Check sheet for the modelled part. Datum: model origin and axes. Units: mm. A direction names the side the tool comes from. Coordinates: 2 decimals unless noted, no trailing zeros. Loops run counter-clockwise (first coordinate to the right, second up) from the corner with the lowest first, then second, coordinate; pieces in that order, holes last.
```python
from build123d import *

# Parameters (mm, degrees)
BOSS_EXTRUDE1_DEPTH   = 7.2
SKETCH1_3_R           = 3.75
SKETCH1_3_R_2         = 1.6
BOSS_EXTRUDE2_DEPTH   = 2
BOSS_EXTRUDE2_2_DEPTH = 2
BOSS_EXTRUDE3_DEPTH   = 2
BOSS_EXTRUDE4_DEPTH   = 7.5
SKETCH3_R             = 3.75
CUT_EXTRUDE6_DEPTH    = 12
BOSS_EXTRUDE5_DEPTH   = 7.5
SKETCH5_R             = 3.75
CUT_EXTRUDE7_DEPTH    = 7.5
SKETCH6_W             = 29.5
SKETCH6_H             = 8.4
BOSS_EXTRUDE6_DEPTH   = 4.3
SKETCH7_W             = 7.5
SKETCH7_H             = 7.2
SKETCH7_W_2           = 16.3
BOSS_EXTRUDE7_DEPTH   = 2
SKETCH8_W             = 10.1
SKETCH8_H             = 2.3
CUT_EXTRUDE8_DEPTH    = 12
SKETCH9_W             = 10.1
SKETCH9_H             = 1.2
BOSS_EXTRUDE8_DEPTH   = 6.4
SKETCH11_W            = 9.1347476
SKETCH11_H            = 5.173710516
BOSS_EXTRUDE11_DEPTH  = 5.5
SKETCH12_R            = 3.106234899
CUT_EXTRUDE10_DEPTH   = 1.5
CUT_EXTRUDE10_DRAFT   = -25
SKETCH13_R            = 3.196774454
CUT_EXTRUDE11_DEPTH   = 1.5
CUT_EXTRUDE11_DRAFT   = -29
SKETCH14_W            = 8.1347476
SKETCH14_H            = 4.5
CUT_EXTRUDE12_DEPTH   = 4.5


# Read off the part's stored shape, not the designer's step: Dome1, Dome2
with BuildPart() as part:
    # Sketch1 → Boss-Extrude1 (new body)
    with BuildSketch(Plane(origin=(0, 0, 0), x_dir=(1, 0, 0), z_dir=(0, 1, 0))):
        Polygon((14.75, 0), (-14.75, 0), (-14.75, -3.75), (-14.75, -6.5), (14.75, -6.5), (14.75, -3.75), align=None)
        Polygon((-14.75, 3.75), (-14.75, 0), (14.75, 0), (14.75, 3.75), (14.75, 6.5), (-14.75, 6.5), align=None)
    extrude(amount=BOSS_EXTRUDE1_DEPTH)



with BuildPart() as body_2:
    # Sketch1<3> → Boss-Extrude2 (new body)
    with BuildSketch(Plane(origin=(0, 0, 0), x_dir=(1, 0, 0), z_dir=(0, 1, 0))):
        with Locations(Location((-18.5, 0, 0), (0, 0, 270))):
            Circle(SKETCH1_3_R)
        with Locations(Location((-18.5, 0, 0), (0, 0, 270))):
            Circle(SKETCH1_3_R_2, mode=Mode.SUBTRACT)
    extrude(amount=BOSS_EXTRUDE2_DEPTH)


with BuildPart() as body_3:
    # Sketch1<3> → Boss-Extrude2 2 (new body)
    with BuildSketch(Plane(origin=(0, 0, 0), x_dir=(1, 0, 0), z_dir=(0, 1, 0))):
        with Locations(Location((18.5, 0, 0), (0, 0, 270))):
            Circle(SKETCH1_3_R)
        with Locations(Location((18.5, 0, 0), (0, 0, 270))):
            Circle(SKETCH1_3_R_2, mode=Mode.SUBTRACT)
    extrude(amount=BOSS_EXTRUDE2_2_DEPTH)


with BuildPart() as part_1:
    add(part.part)

    add(body_2.part)  # Boss-Extrude3 merges body 2

    add(body_3.part)  # Boss-Extrude3 merges body 3
    # Sketch1<4> → Boss-Extrude3 (add)
    with BuildSketch(Plane(origin=(0, 0, 0), x_dir=(1, 0, 0), z_dir=(0, 1, 0))):
        with BuildLine():
            Line((-14.75, -3.75), (-14.75, 0))
            ThreePointArc((-14.75, 0), (-15.848349571, -2.651650429), (-18.5, -3.75))
            Line((-18.5, -3.75), (-14.75, -3.75))
        make_face()
        with BuildLine():
            Line((-14.75, 0), (-14.75, 3.75))
            Line((-14.75, 3.75), (-18.5, 3.75))
            ThreePointArc((-18.5, 3.75), (-15.848349571, 2.651650429), (-14.75, 0))
        make_face()
        with BuildLine():
            Line((18.5, 3.75), (14.75, 3.75))
            Line((14.75, 3.75), (14.75, 0))
            ThreePointArc((14.75, 0), (15.848349571, 2.651650429), (18.5, 3.75))
        make_face()
        with BuildLine():
            ThreePointArc((18.5, -3.75), (15.848349571, -2.651650429), (14.75, 0))
            Line((14.75, 0), (14.75, -3.75))
            Line((14.75, -3.75), (18.5, -3.75))
        make_face()
    extrude(amount=BOSS_EXTRUDE3_DEPTH)

    # Sketch2 → Boss-Extrude4 (add)
    with BuildSketch(Plane.XY.offset(3.75)):
        Polygon((18.5, 2), (14.75, 2), (14.75, 5.75), align=None)
    extrude(amount=-BOSS_EXTRUDE4_DEPTH)

    # Sketch3 → Cut-Extrude6 (cut)
    with BuildSketch(Plane(origin=(0, 2, 0), x_dir=(1, 0, 0), z_dir=(0, 1, 0))):
        with Locations((18.5, 0)):
            Circle(SKETCH3_R)
    extrude(amount=CUT_EXTRUDE6_DEPTH, mode=Mode.SUBTRACT)

    # Sketch4 → Boss-Extrude5 (add)
    with BuildSketch(Plane.XY.offset(3.75)):
        Polygon((-14.75, 5.75), (-18.5, 2), (-14.75, 2), align=None)
    extrude(amount=-BOSS_EXTRUDE5_DEPTH)

    # Sketch5 → Cut-Extrude7 (cut)
    with BuildSketch(Plane(origin=(0, 2, 0), x_dir=(1, 0, 0), z_dir=(0, 1, 0))):
        with Locations((-18.5, 0)):
            Circle(SKETCH5_R)
    extrude(amount=CUT_EXTRUDE7_DEPTH, mode=Mode.SUBTRACT)

    # Sketch6 → Boss-Extrude6 (add)
    with BuildSketch(Plane(origin=(0, 7.2, 0), x_dir=(1, 0, 0), z_dir=(0, 1, 0))):
        Rectangle(SKETCH6_W, SKETCH6_H)
    extrude(amount=BOSS_EXTRUDE6_DEPTH)

    # Sketch7 → Boss-Extrude7 (add)
    with BuildSketch(Plane(origin=(0, 11.5, 0), x_dir=(1, 0, 0), z_dir=(0, 1, 0))):
        with Locations((-10.25, 0)):
            Rectangle(SKETCH7_W, SKETCH7_H)
        with Locations((5.8, 0)):
            Rectangle(SKETCH7_W_2, SKETCH7_H)
    extrude(amount=BOSS_EXTRUDE7_DEPTH)

    # Sketch8 → Cut-Extrude8 (cut)
    with BuildSketch(Plane(origin=(0, 7.2, 0), x_dir=(1, 0, 0), z_dir=(0, 1, 0))):
        with Locations((0.003829246, -5.35)):
            Rectangle(SKETCH8_W, SKETCH8_H)
    extrude(amount=-CUT_EXTRUDE8_DEPTH, mode=Mode.SUBTRACT)

    # Sketch9 → Boss-Extrude8 (add)
    with BuildSketch(Plane.XY.offset(4.2)):
        with Locations((0.003829246, 3.9)):
            Rectangle(SKETCH9_W, SKETCH9_H)
    extrude(amount=BOSS_EXTRUDE8_DEPTH)

    # Sketch11 → Boss-Extrude11 (add)
    with BuildSketch(Plane(origin=(0, 4.5, 0), x_dir=(1, 0, 0), z_dir=(0, 1, 0))):
        with Locations((0.014014126, -7.894862881)):
            Rectangle(SKETCH11_W, SKETCH11_H)
    extrude(amount=BOSS_EXTRUDE11_DEPTH)


with BuildPart() as cut_extrude10_tool:
    # Sketch12 → Cut-Extrude10 (with draft: the straight prism first)
    with BuildSketch(Plane(origin=(0, 13.5, 0), x_dir=(1, 0, 0), z_dir=(0, 1, 0))):
        with Locations((-10.25, 0)):
            Circle(SKETCH12_R)
    extrude(amount=-CUT_EXTRUDE10_DEPTH)
    # Cut-Extrude10: the draft: its side faces are tilted about the plane it starts from
    cut_extrude10_sides = [cut_extrude10_tool.faces().sort_by_distance(p)[0] for p in [
        (-13.356234899, 12.75, 0),
    ]]
    draft(cut_extrude10_sides, Plane(origin=(0, 13.5, 0), x_dir=(1, 0, 0), z_dir=(0, 1, 0)), CUT_EXTRUDE10_DRAFT)


with BuildPart() as part_2:
    add(part_1.part)

    # Cut-Extrude10: cut by cut_extrude10_tool
    add(cut_extrude10_tool.part, mode=Mode.SUBTRACT)


with BuildPart() as cut_extrude11_tool:
    # Sketch13 → Cut-Extrude11 (with draft: the straight prism first)
    with BuildSketch(Plane(origin=(0, 13.5, 0), x_dir=(1, 0, 0), z_dir=(0, 1, 0))):
        with Locations((9.516994158, 0)):
            Circle(SKETCH13_R)
    extrude(amount=-CUT_EXTRUDE11_DEPTH)
    # Cut-Extrude11: the draft: its side faces are tilted about the plane it starts from
    cut_extrude11_sides = [cut_extrude11_tool.faces().sort_by_distance(p)[0] for p in [
        (6.320219704, 12.75, 0),
    ]]
    draft(cut_extrude11_sides, Plane(origin=(0, 13.5, 0), x_dir=(1, 0, 0), z_dir=(0, 1, 0)), CUT_EXTRUDE11_DRAFT)


with BuildPart() as part_3:
    add(part_2.part)

    # Cut-Extrude11: cut by cut_extrude11_tool
    add(cut_extrude11_tool.part, mode=Mode.SUBTRACT)

    # Dome1 outline → Dome1 (revolve)
    with BuildSketch(Plane(origin=(-10.25, 0, 0), x_dir=(1, 0, 0), z_dir=(0, 0, 1))):
        with BuildLine():
            Line((0, 12), (2.406773413, 11.999999998))
            ThreePointArc((2.406773413, 11.999999998), (1.417970228, 13.094302608), (0, 13.5))
            Line((0, 13.5), (0, 12))
        make_face()
    revolve(axis=Axis((-10.25, 0, 0), (0, 1, 0)))

    # Dome2 outline → Dome2 (revolve)
    with BuildSketch(Plane(origin=(9.516994158, 0, 0), x_dir=(1, 0, 0), z_dir=(0, 0, 1))):
        with BuildLine():
            Line((0, 12), (2.365310878, 11.999999998))
            ThreePointArc((2.365310878, 11.999999998), (1.400419183, 13.093385967), (0, 13.5))
            Line((0, 13.5), (0, 12))
        make_face()
    revolve(axis=Axis((9.516994158, 0, 0), (0, 1, 0)))

    # Sketch14 → Cut-Extrude12 (cut)
    with BuildSketch(Plane.XY.offset(10.481718139)):
        with Locations((0.014014126, 7.25)):
            Rectangle(SKETCH14_W, SKETCH14_H)
    extrude(amount=-CUT_EXTRUDE12_DEPTH, mode=Mode.SUBTRACT)


solid = part_3.part
```
1) Section check C-C on x = -3.5. Enter the section's corners in (y, z), plus the area to 3 significant figures.
Answer sheet:
outline: (0, -6.5) - (7.2, -6.5) - (7.2, -4.2) - (11.5, -4.2) - (11.5, 4.2) - (4.5, 4.2) - (4.5, 5.31) - (10, 5.31) - (10, 10.48) - (9.5, 10.48) - (9.5, 5.98) - (5, 5.98) - (5, 10.48) - (4.5, 10.48) - (4.5, 10.6) - (3.3, 10.6) - (3.3, 4.2) - (0, 4.2) - close
area: 129 mm2
2) Section check B-B on y = 8. Enter the section's corners in (x, z), plus the area to 3 significant figures.
Answer sheet:
outline: (-14.75, -4.2) - (14.75, -4.2) - (14.75, 4.2) - (-14.75, 4.2) - close; (-4.55, 5.31) - (4.58, 5.31) - (4.58, 10.48) - (4.08, 10.48) - (4.08, 5.98) - (-4.05, 5.98) - (-4.05, 10.48) - (-4.55, 10.48) - close
area: 258 mm2
3) Section check D-D on x = 15.5. Enter the section's corners in (y, z).
Answer sheet:
outline: (0, -3.75) - (5, -3.75) - (5, -2.25) - (2, -2.25) - (2, 2.25) - (5, 2.25) - (5, 3.75) - (0, 3.75) - close
4) Section check A-A on x = -10.25. Enter the section's corners in (y, z), plus the area to 3 significant figures.
Answer sheet:
outline: (0, -6.5) - (7.2, -6.5) - (7.2, -4.2) - (11.5, -4.2) - (11.5, -3.6) - (13.5, -3.6) - (13.5, -3.11) - (12, -2.41) arc R2.68 ccw to (12, 2.41) - (13.5, 3.11) - (13.5, 3.6) - (11.5, 3.6) - (11.5, 4.2) - (7.2, 4.2) - (7.2, 6.5) - (0, 6.5) - close
area: 141 mm2
5) Depth check by flat-ended pin: pin 1 (3.5 mm diameter, centred on x = -10.5, y = 2.5, fed in from +Z); pin 2 (4 mm diameter, centred on y = 9.5, z = 0.5, fed in from +X); pin 3 (3 mm diameter, centred on x = 18.5, z = 0, fed in from +Y); pin 4 (3 mm diameter, centred on x = -16.5, y = 4, fed in from +Z). Enter the tip coordinate at first touch or a pass-through.
Answer sheet:
pin 1: stops at z = 6.5
pin 2: stops at x = 14.75
pin 3: passes through
pin 4: stops at z = 3.75
6) Set-up check for faces 1 (the flat face through (13.95, 12, 0)), 2 (the flat face through (-6.5, 12, 0)), 3 (the flat face through (-10, 7.2, 5)): record each of +Z, -Z, +X, -X, +Y, -Y from which the full face is reachable in a straight line by a thin tool's end or side.
Answer sheet:
face 1: +Z, -Z, +X, +Y
face 2: +Z, -Z, +Y
face 3: +Z, -X, +Y
7) Scan lines: line 1 (X direction, y = 1.25, z = 0); line 2 (Y direction, x = 1, z = 6.5); line 3 (Z direction, x = 1.5, y = 9). Record each from-to range of solid material in increasing order.
Answer sheet:
line 1: x = -22.25 to -20.1, -16.9 to 16.9, 20.1 to 22.25
line 2: y = 3.3 to 5, 9.5 to 10
line 3: z = -4.2 to 4.2, 5.31 to 5.98
8) Mould release check, pull along Z, two halves, no side actions. Record for faces 4 (the cylindrical face through (-14.75, 3.43, 0.08)), 5 (the flat face through (0, 2, 4.2)), 6 (the flat face through (-4.553, 7, 8)): +Z half, -Z half, draft (parallel to the pull), parting line (faces both ways), or undercut.
Answer sheet:
face 4: undercut
face 5: +Z half
face 6: draft
